from build123d import *

# Parameters (mm, degrees)
SKETCH1_W           = 12.7
SKETCH1_H           = 190.5
BOSS_EXTRUDE1_DEPTH = 5.08
SKETCH5_W           = 3.175
SKETCH5_H           = 5.08
SKETCH5_W_2         = 11.1125
BOSS_EXTRUDE2_DEPTH = 190.5
SKETCH6_R           = 0.8255
CUT_EXTRUDE1_DEPTH  = 97.432752618
SKETCH7_W           = 1.5875
SKETCH7_H           = 5.08
BOSS_EXTRUDE3_DEPTH = 12.7


with BuildPart() as part:
    # Sketch1 → Boss-Extrude1 (new body)
    with BuildSketch(Plane.XY):
        Rectangle(SKETCH1_W, SKETCH1_H)
    extrude(amount=BOSS_EXTRUDE1_DEPTH)

    # Cut-Loft1: read off the stored shape, not the designer's step
    # Cut-Loft1: loft between two sections, ruled curve by curve
    cut_loft1_from = [
        Edge.make_bspline([(6.35, -92.71, 0.635), (6.35, -92.880627047, 0.635), (6.35, -93.190295538, 0.679451635), (6.35, -93.580426831, 0.829875615), (6.35, -93.904017113, 1.040042177), (6.35, -94.252532736, 1.378638842), (6.35, -94.539016945, 1.880682246), (6.35, -94.652993182, 2.54), (6.35, -94.539016945, 3.199317754), (6.35, -94.252532736, 3.701361158), (6.35, -93.904017113, 4.039957823), (6.35, -93.580426831, 4.250124385), (6.35, -93.190295538, 4.400548365), (6.35, -92.880627047, 4.445), (6.35, -92.100030361, 4.445), (6.35, -90.729103522, 4.445), (6.35, -87.9475, 4.445), (6.35, -85.165896478, 4.445), (6.35, -83.794969639, 4.445), (6.35, -83.185, 4.445)], [0, 0, 0, 0, 0.033003864, 0.066007727, 0.099011591, 0.132015455, 0.198023182, 0.264030909, 0.330038636, 0.396046364, 0.429050227, 0.462054091, 0.495057954, 0.528061818, 0.528061818, 0.646046364, 0.764030909, 0.882015455, 1, 1, 1, 1], 3),
        Edge.make_bspline([(6.35, -83.185, 4.445), (6.35, -82.922150477, 4.445), (6.35, -82.421175953, 4.339900308), (6.35, -81.805369524, 3.916723034), (6.35, -81.386700238, 3.309409446), (6.35, -81.226649881, 2.54), (6.35, -81.386700238, 1.770590554), (6.35, -81.805369524, 1.163276966), (6.35, -82.421175953, 0.740099692), (6.35, -82.922150477, 0.635), (6.35, -83.185, 0.635)], [0, 0, 0, 0, 0.125, 0.25, 0.375, 0.5, 0.625, 0.75, 0.875, 1, 1, 1, 1], 3),
        Edge.make_line((6.35, -92.71, 0.635), (6.35, -83.185, 0.635)),
    ]
    cut_loft1_to = [
        Edge.make_bspline([(-6.35, -92.71, 0.635), (-6.35, -92.81076887, 0.635), (-6.35, -93.018481978, 0.65100327), (-6.35, -93.339219021, 0.731183475), (-6.35, -93.659764721, 0.875704473), (-6.35, -94.064204291, 1.159019535), (-6.35, -94.484151999, 1.692137872), (-6.35, -94.680912476, 2.54), (-6.35, -94.484151999, 3.387862128), (-6.35, -94.064204291, 3.920980465), (-6.35, -93.659764721, 4.204295527), (-6.35, -93.339219021, 4.348816525), (-6.35, -93.018481978, 4.42899673), (-6.35, -92.81076887, 4.445), (-6.35, -92.349764316, 4.445), (-6.35, -91.828550912, 4.445), (-6.35, -91.1225, 4.445), (-6.35, -90.416449088, 4.445), (-6.35, -89.895235684, 4.445), (-6.35, -89.535, 4.445)], [0, 0, 0, 0, 0.033003864, 0.066007727, 0.099011591, 0.132015455, 0.198023182, 0.264030909, 0.330038636, 0.396046364, 0.429050227, 0.462054091, 0.495057954, 0.528061818, 0.528061818, 0.646046364, 0.764030909, 0.882015455, 1, 1, 1, 1], 3),
        Edge.make_bspline([(-6.35, -89.535, 4.445), (-6.35, -89.535, 4.28625), (-6.35, -89.535, 3.96875), (-6.35, -89.535, 3.4925), (-6.35, -89.535, 3.01625), (-6.35, -89.535, 2.54), (-6.35, -89.535, 2.06375), (-6.35, -89.535, 1.5875), (-6.35, -89.535, 1.11125), (-6.35, -89.535, 0.79375), (-6.35, -89.535, 0.635)], [0, 0, 0, 0, 0.125, 0.25, 0.375, 0.5, 0.625, 0.75, 0.875, 1, 1, 1, 1], 3),
        Edge.make_line((-6.35, -92.71, 0.635), (-6.35, -89.535, 0.635)),
    ]
    cut_loft1 = Solid(Shell([*[Face.make_surface_from_curves(cut_loft1_from[k], cut_loft1_to[k]) for k in range(3)], Face(Wire(cut_loft1_from)), Face(Wire(cut_loft1_to))]))
    add(cut_loft1, mode=Mode.SUBTRACT)

    # Sketch5 → Boss-Extrude2 (add)
    with BuildSketch(Plane.XZ.offset(95.25)):
        with Locations((3.175, 7.62)):
            Rectangle(SKETCH5_W, SKETCH5_H)
        with Locations((-0.79375, -2.54)):
            Rectangle(SKETCH5_W_2, SKETCH5_H)
    extrude(amount=-BOSS_EXTRUDE2_DEPTH)

    # Sketch6 → Cut-Extrude1 (cut, through all)
    with BuildSketch(Plane(origin=(4.7625, 0, 0), x_dir=(0, 0, -1), z_dir=(1, 0, 0))):
        with Locations((-7.62, -92.71)):
            Circle(SKETCH6_R)
    extrude(amount=-CUT_EXTRUDE1_DEPTH, mode=Mode.SUBTRACT)

    # Sketch7 → Boss-Extrude3 (add)
    with BuildSketch(Plane(origin=(0, 95.25, 0), x_dir=(1, 0, 0), z_dir=(0, 1, 0))):
        with Locations((5.55625, 2.54)):
            Rectangle(SKETCH7_W, SKETCH7_H)
        with Locations((5.55625, -7.62)):
            Rectangle(SKETCH7_W, SKETCH7_H)
    extrude(amount=-BOSS_EXTRUDE3_DEPTH)


solid = part.part
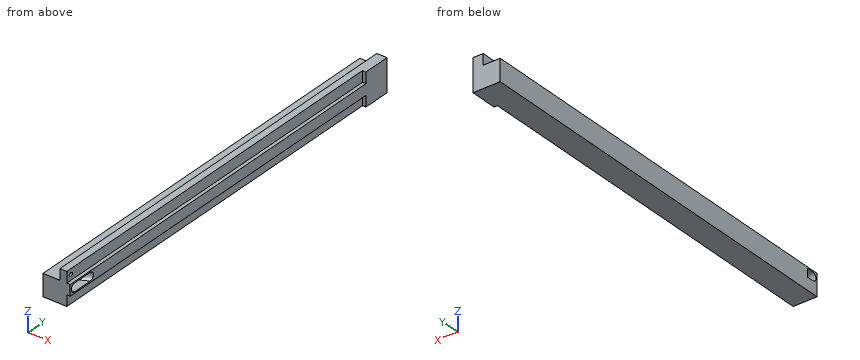
Design review of the part built by this model. Coordinates are the model's own, in mm. Give positions to 0.01 mm unless a question says otherwise; leave off trailing zeros. Loops run counter-clockwise (first coordinate to the right, second up) from the corner with the lowest first, then second, coordinate; pieces in that order, holes last. Notation, with made-up numbers: (-21, 17) - (1, 17) arc R29 ccw to (1, 46) - close; hole circle Ø8 at (-34, 61). An arc over 180 degrees is marked (long way). Write item = value, one per line.
1) To check wall thickness, follow line 1 (Z direction, x = 2.35, y = -92.71) (1 decimal); line 2 (Y direction, x = 3.1, z = 7.62); line 3 (X direction, y = -25, z = 8.75). State the ranges of each line that lie inside material, in increasing order.
Result sheet:
line_1 = -5.1 to 0.6, 4.4 to 6.8, 8.4 to 10.2
line_2 = -95.25 to -93.54, -91.88 to 95.25
line_3 = 1.59 to 4.76
2) Take a section at A-A on y = -57. State the section outline as (x, z) points, and give its area (3 significant figures).
Result sheet:
outline = (-6.35, -5.08) - (4.76, -5.08) - (4.76, 0) - (6.35, 0) - (6.35, 5.08) - (4.76, 5.08) - (4.76, 10.16) - (1.59, 10.16) - (1.59, 5.08) - (-6.35, 5.08) - close
area = 137 mm2
3) Clearance check with flat-ended pins moving along their axes: pin 1 Ø4 at (y, z) = (-31.5, 7.5) entering from -X; pin 2 Ø1.3 at (x, z) = (5.5, 7.5) entering from -Y; pin 3 Ø0.8 at (x, y) = (5.5, -14) entering from +Z. State where each tip first meets the part, or that it passes through.
Result sheet:
pin_1 = 1.59
pin_2 = 82.55
pin_3 = 5.08
4) Take a section at B-B on z = -2.75. State the section outline as (x, y) points.
Result sheet:
outline = (-6.35, -95.25) - (4.76, -95.25) - (4.76, 82.55) - (6.35, 82.55) - (6.35, 95.25) - (-6.35, 95.25) - close
